from build123d import *

# Parameters (mm, degrees)
F0_W      = 400
F0_H      = 400
F1_DEPTH  = 400
F2_W      = 300
F2_H      = 350
F3_DEPTH  = 400.001
F4_W      = 300
F4_H      = 350
F5_DEPTH  = 400.001
F10_W     = 400
F10_H     = 300
F11_DEPTH = 50
F12_W     = 300
F12_H     = 300
F13_DEPTH = 122.9991389297
F15_DEPTH = 50
F17_DEPTH = 50
F19_DEPTH = 180


with BuildPart() as f1:
    # F0 (on Top) → F1 (new body)
    with BuildSketch(Plane.XY):
        Rectangle(F0_W, F0_H)
    extrude(amount=F1_DEPTH)

    # F2 (on face) → F3 (cut, through all)
    with BuildSketch(Plane.XZ.offset(200)):
        with Locations((0, 175)):
            Rectangle(F2_W, F2_H)
    extrude(amount=-F3_DEPTH, mode=Mode.SUBTRACT)

    # F4 (on face) → F5 (cut, through all)
    with BuildSketch(Plane.YZ.offset(200)):
        with Locations((0, 175)):
            Rectangle(F4_W, F4_H)
    extrude(amount=-F5_DEPTH, mode=Mode.SUBTRACT)



with BuildPart() as f11:
    # F10 (on line) → F11 (new body)
    with BuildSketch(Plane(origin=(-156.2324219098, 0, -16.4206892285), x_dir=(0, -1, 0), z_dir=(-0.9945218954, 0, -0.1045284633))):
        with Locations((0, 568.7144508008)):
            Rectangle(F10_W, F10_H)
    extrude(amount=-F11_DEPTH)

    # F12 (on face) → F13 (cut, through all)
    with BuildSketch(Plane(origin=(-106.5063271414, 0, -11.1942660652), x_dir=(0, 1, 0), z_dir=(0.9945218954, 0, 0.1045284633))):
        with Locations((0, 568.7144508008)):
            Rectangle(F12_W, F12_H)
    extrude(amount=-F13_DEPTH, mode=Mode.SUBTRACT)


with BuildPart() as f1_1:
    add(f1.part)

    add(f11.part)  # F15 merges F11
    # F14 (on face) → F15 (join)
    with BuildSketch(Plane(origin=(0, 200, 0), x_dir=(-1, 0, 0), z_dir=(0, 1, 0))):
        Polygon((149.7245860218, 400), (200, 400), (150.2739052316, 405.2264231634), align=None)
    extrude(amount=-F15_DEPTH)

    # F16 (on face) → F17 (join)
    with BuildSketch(Plane.XZ.offset(200)):
        Polygon((-150.2739052316, 405.2264231634), (-200, 400), (-149.7245860218, 400), align=None)
    extrude(amount=-F17_DEPTH)

    # F18 (on face) → F19 (join)
    with BuildSketch(Plane(origin=(-75.1261170705, 0, 714.777257839), x_dir=(0.9945218954, 0, 0.1045284633), z_dir=(-0.1045284633, 0, 0.9945218954))):
        with BuildLine():
            ThreePointArc((-107.0929937666, -150), (-167.7233901133, 0), (-107.0929937666, 150))
            Line((-107.0929937666, 150), (-133.8813907821, 150))
            ThreePointArc((-133.8813907821, 150), (-187.7233901133, 0), (-133.8813907821, -150))
            Line((-133.8813907821, -150), (-107.0929937666, -150))
        make_face()
    extrude(amount=-F19_DEPTH)


solid = f1_1.part
Source: CAD feature listing. Evaluate the final solid. Frame: model axes, mm. A direction names the side the tool comes from. Round coordinates to 2 decimals unless told otherwise and drop trailing zeros. Loops run counter-clockwise (first coordinate to the right, second up) from the corner with the lowest first, then second, coordinate; pieces in that order, holes last. Notation, with made-up numbers: (56.25, 21) - (80.25, 21) arc R29 ccw to (80.25, 46) - close; hole circle Ø10 at (-22.75, 72.5). An arc over 180 degrees is marked (long way). Write item = value, one per line. Start each with the question number.
(1) Pull-direction query (X, two-part tool) for faces 1 (the face through (3, -3, 350)), 2 (the face through (200, -1, 362)), 3 (the face through (150, -175, 173)), 4 (the face through (175, -175, 0)); classes: +X half, -X half, draft (parallel to the pull), parting line (faces both ways), or undercut.
(2) Section query C-C, the plane z = 427. Output: boundary loops of the cut face in (x, y), plus the area to 3 significant figures.
(3) Ray query, line 1 along Y through (x, z) = (-199, 95); line 2 along Z through (x, y) = (23.5, -70.5). Return the intervals inside material, ascending. Write a range as from..to.
(4) Section query D-D, the plane x = 132.5. Output: boundary loops of the cut face in (y, z), plus the area to 3 significant figures.
(5) Pin query (flat end, axial travel): pin 1 (2 mm diameter, centred on x = 110.5, y = -152, fed in from +Z); pin 2 (10 mm diameter, centred on y = 144, z = 82.5, fed in from +X); pin 3 (25 mm diameter, centred on y = -165, z = 93, fed in from -X); pin 4 (1.5 mm diameter, centred on y = -146.5, z = 625, fed in from +X). Return the tip coordinate at first contact, or that it passes through.
(6) Section query B-B, the plane y = -27.5. Output: boundary loops of the cut face in (x, z).
(7) Section query A-A, the plane z = 86. Output: boundary loops of the cut face in (x, y).
(8) Set-up query: faces 5 (the face through (-223.89, -10.41, 518.15)), 6 (the face through (-215.9, 175.35, 551.27)), 7 (the face through (-200, -1, 362)). Return all of +Z, -Z, +X, -X, +Y, -Y with unobstructed straight access to the full face (end or side cutting, diameter ignored); none if empty.
Conclusion:
q1.face_1 = undercut
q1.face_2 = +X half
q1.face_3 = undercut
q1.face_4 = draft
q2.outline = (-202.84, -200) - (-152.56, -200) - (-152.56, -150) - (-202.84, -150) - close; (-202.84, 150) - (-152.56, 150) - (-152.56, 200) - (-202.84, 200) - close
q2.area = 5,030 mm2
q3.line_1 = -200..-150, 150..200
q3.line_2 = 350..400
q4.outline = (-200, 350) - (200, 350) - (200, 400) - (-200, 400) - close
q4.area = 20,000 mm2
q5.pin_1 = 400
q5.pin_2 = through
q5.pin_3 = -200
q5.pin_4 = -175.99
q6.outline = (-260.22, 695.32) - (-241.41, 516.31) - (-221.37, 518.42) - (-240.18, 697.43) - close; (-200, 350) - (200, 350) - (200, 400) - (-200, 400) - close
q7.outline = (-200, -200) - (-150, -200) - (-150, -150) - (-200, -150) - close; (-200, 150) - (-150, 150) - (-150, 200) - (-200, 200) - close; (150, -200) - (200, -200) - (200, -150) - (150, -150) - close; (150, 150) - (200, 150) - (200, 200) - (150, 200) - close
q8.face_5 = +X
q8.face_6 = -Z, -X, +Y
q8.face_7 = -Z, -X, +Y, -Y
